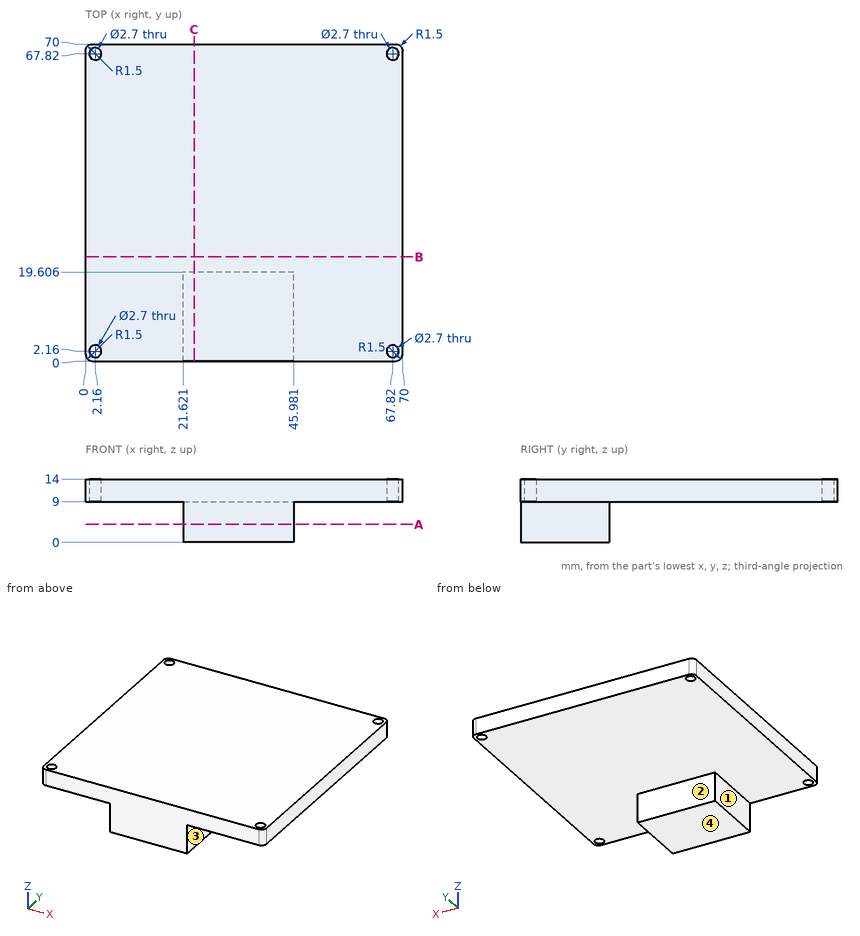
Could you check a few things on this drawing? It's one solid part, dimensions in mm from its lowest x, y, z. A direction names the side the tool comes from. Give positions to 0.01 mm unless a question says otherwise; leave off trailing zeros. Loops run counter-clockwise (first coordinate to the right, second up) from the corner with the lowest first, then second, coordinate; pieces in that order, holes last. Notation, with made-up numbers: M 7.5,-24 L 58.5,-24 A13 ccw 58.5,-5 Z; hole C 18,57 d4. An arc over 180 degrees is marked long. Answer as a JSON object with one key per item and string values.
Q1. Suppose I cut it at C-C, the plane x = 24. List the corners of the cut face in (y, z) for me.
Values found:
{"outline": "M 0,0 L 19.61,0 L 19.61,9 L 70,9 L 70,14 L 0,14 Z"}
Q2. If I drill on probe 1 along Y at (x, z) = (67.82, 13); probe 2 along Z at (x, y) = (10.5, 43); probe 3 along X at (y, z) = (14, 2.25), over which ranges is the centre line in solid material (lowest first)? Write a range as [from, to].
Values found:
{"probe 1": "y = [0, 0.81], [3.51, 66.47], [69.17, 70]", "probe 2": "z = [9, 14]", "probe 3": "x = [21.62, 45.98]"}
Q3. Suppose I cut it at A-A, the plane z = 4. List the corners of the cut face in (x, y) for me.
Values found:
{"outline": "M 21.62,0 L 45.98,0 L 45.98,19.61 L 21.62,19.61 Z"}
Q4. For P1, Ø4, axis at x = 38.5, y = 39.5, coming from the -Z side; P2, Ø2.5, axis at x = 36.5, z = 3.5, coming from the +Y side; P3, Ø2.5, axis at y = 6, z = 3, coming from the -X side, each with a flat end and sliding along its axis, tell me the tip position at first contact or that it passes through.
Values found:
{"P1": "stops at z = 9", "P2": "stops at y = 19.61", "P3": "stops at x = 21.62"}
Q5. Suppose I cut it at B-B, the plane y = 23. List the corners of the cut face in (x, z) for me, plus the area to 3 significant figures.
Values found:
{"outline": "M 0,9 L 70,9 L 70,14 L 0,14 Z", "area": "350 mm²"}
Q6. For the marked faces 1, 2, 3 and 4, which set-ups out of +Z, -Z, +X, -X, +Y, -Y let a thin tool reach every point of the face, with its end or its side?
Values found:
{"face 1": "-Z, -X, +Y, -Y", "face 2": "-Z, +X, -X, +Y", "face 3": "-Z, +X, +Y, -Y", "face 4": "-Z, +X, -X, +Y, -Y"}
